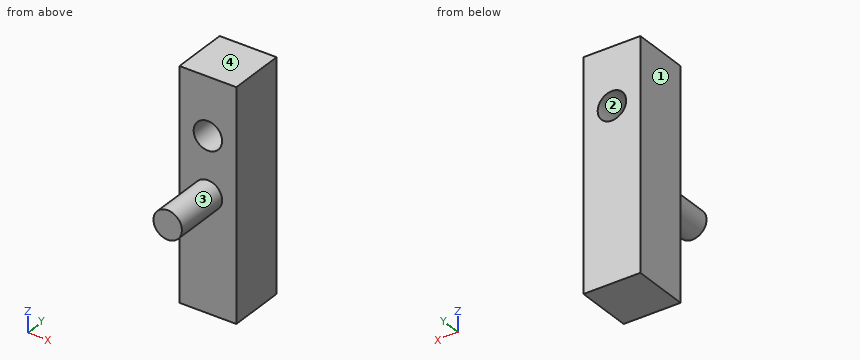
Autodesk Inventor part; units mm, degrees
ref_plane "YZ Plane" through (0, 0, 0) normal (1, 0, 0) x (0, 1, 0)
ref_plane "XZ Plane" through (0, 0, 0) normal (0, 1, 0) x (-1, 0, 0)
ref_plane "XY Plane" through (0, 0, 0) normal (0, 0, 1) x (1, 0, 0)
sketch "Sketch1" plane through (0, 0, 0) normal (0, 1, 0) x (-1, 0, 0)
  circle A0 centre (0, 0) radius 6.35
  dimension "d0" = 12.7
extrude "Extrusion1" add sketch "Sketch1" along normal blind 25.4
sketch "Sketch2" plane through (0, 25.4, 0) normal (0, 1, 0) x (1, 0, 0)
  line L0 (12.7, 50.8) -> (-12.7, 50.8)
  line L1 (-12.7, 50.8) -> (-12.7, -50.8)
  line L2 (-12.7, -50.8) -> (12.7, -50.8)
  line L3 (12.7, -50.8) -> (12.7, 50.8)
  line L4 (12.7, 50.8) -> (-12.7, -50.8) construction
  line L5 (-12.7, 50.8) -> (12.7, -50.8) construction
  point P0 (0, 0)
  dimension "d3" = 101.6
  dimension "d4" = 25.4
extrude "Extrusion2" add sketch "Sketch2" along normal blind 25.4
sketch "Sketch3" plane through (0, 50.8, 0) normal (0, 1, 0) x (1, 0, 0)
  circle A0 centre (0, -25.4) radius 6.35
  line L0 (-12.7, -50.8) -> (12.7, -50.8)
  point P0 (0, 0)
  dimension "d7" = 25.4
  dimension "d8" = 12.7
extrude "Extrusion3" cut sketch "Sketch3" against normal through all
properties part number "knuckle"
Geometry check sheet. Reference: the model listing, model coordinates, mm. Face numbers are marked on the shaded views. Round coordinates to 2 decimals unless told otherwise and drop trailing zeros. Order: outer loops, then holes, each group sorted by start corner. A loop starts at its lowest first (then second) coordinate and runs counter-clockwise, first axis right, second up. Notation, with made-up numbers: M 70,71 L 121,71 A30 ccw 121,108 Z; hole C 31,6.25 d1. An arc over 180 degrees is marked long. Answer as CSV lines item,"result".
1) Sectioned sample at B-B on z = 0. Record the cut outline in (x, y).
Entries:
outline,"M -12.7,25.4 L -6.35,25.4 L -6.35,0 L 6.35,0 L 6.35,25.4 L 12.7,25.4 L 12.7,50.8 L -12.7,50.8 Z"
2) Thickness scan on probe 1 along Z at (x, y) = (0, 32.5); probe 2 along X at (y, z) = (41.25, 25.4); probe 3 along Y at (x, z) = (8, -1.5). Record the ranges inside material, lowest first. Write a range as [from, to].
Entries:
probe 1,"[-50.8, 19.05], [31.75, 50.8]"
probe 2,"[-12.7, -6.35], [6.35, 12.7]"
probe 3,"[25.4, 50.8]"
3) Sectioned sample at A-A on z = 25.4. Record the cut outline in (x, y).
Entries:
outline,"M -12.7,25.4 L -6.35,25.4 L -6.35,50.8 L -12.7,50.8 Z; M 6.35,25.4 L 12.7,25.4 L 12.7,50.8 L 6.35,50.8 Z"
4) Gauge pin test, flat ends, axial feed: pin 1 Ø4 at (x, z) = (-7, -14) entering from -Y; pin 2 Ø2 at (y, z) = (13, 5.5) entering from +X; pin 3 Ø3 at (y, z) = (22, -21) entering from -X; pin 4 Ø3 at (x, y) = (-3, 23.5) entering from -Z. Record the tip position at first contact, or that the pin passes through.
Entries:
pin 1,"y = 25.4"
pin 2,"x = 4.48"
pin 3,"through"
pin 4,"z = -6.17"
5) Sectioned sample at D-D on x = -1. Record the cut outline in (y, z).
Entries:
outline,"M 0,-6.27 L 25.4,-6.27 L 25.4,-50.8 L 50.8,-50.8 L 50.8,19.13 L 25.4,19.13 L 25.4,6.27 L 0,6.27 Z; M 25.4,31.67 L 50.8,31.67 L 50.8,50.8 L 25.4,50.8 Z"
6) Sectioned sample at C-C on y = 36. Record the cut outline in (x, z).
Entries:
outline,"M -12.7,-50.8 L 12.7,-50.8 L 12.7,50.8 L -12.7,50.8 Z; hole C 0,25.4 d12.7"
7) Mould release check, pull along X, two halves, no side actions. Record for the marked faces 1, 2, 3 and 4: +X half, -X half, draft (parallel to the pull), parting line (faces both ways), or undercut.
Entries:
face 1,"-X half"
face 2,"undercut"
face 3,"parting line"
face 4,"draft"
